Verification items for the finished model (mm, model axes). Face numbers are marked on the shaded views. A direction names the side the tool comes from. Coordinates: 2 decimals unless noted, no trailing zeros. Order: outer loops, then holes, each group sorted by start corner. A loop starts at its lowest first (then second) coordinate and runs counter-clockwise, first axis right, second up. Notation, with made-up numbers: M 70,7 L 115,7 A9 ccw 115,20 Z; hole C -32.75,19.5 d5. An arc over 180 degrees is marked long. Use one line per item in the form item = value. Start each with the question number.
```python
from build123d import *
from build123d.topology import SkipClean

# Parameters (mm, degrees)
BASE_EXTRUDE_DEPTH  = 5.76
SKETCH2_R           = 2.65
BOSS_EXTRUDE1_DEPTH = 9.45
CUT_EXTRUDE3_DEPTH  = 53.449290987
SKETCH4_R           = 1.37
BOSS_EXTRUDE2_DEPTH = 2.64
BOSS_EXTRUDE2_DRAFT = -1
SKETCH7_R           = 1.15
CUT_EXTRUDE4_DEPTH  = 11.09
CUT_EXTRUDE5_DEPTH  = 53.988618848
CUT_EXTRUDE6_START  = -3.76
CUT_EXTRUDE6_DEPTH  = 3.76
BOSS_EXTRUDE3_DEPTH = 1.65
SKETCH11_W          = 10.1
SKETCH11_H          = 3.76
CUT_EXTRUDE7_DEPTH  = 1.5
SKETCH12_W          = 10.1
SKETCH12_H          = 1.65
CUT_EXTRUDE8_DEPTH  = 1.5
BOSS_EXTRUDE4_DEPTH = 3.76
FILLET1_R           = 0.7
BOSS_EXTRUDE5_START = -3.76
BOSS_EXTRUDE5_DEPTH = 5.18
FILLET5_R           = 0.685
BOSS_EXTRUDE6_DEPTH = 3.48
BOSS_EXTRUDE7_START = -1.26
BOSS_EXTRUDE7_DEPTH = 1.26
BOSS_EXTRUDE8_DEPTH = 4
SKETCH18_W          = 2
SKETCH18_H          = 4.75
CUT_EXTRUDE9_DEPTH  = 48.255056695
FILLET2_R           = 1
SKETCH21_R          = 1.46
CUT_EXTRUDE13_DEPTH = 6.58


with BuildPart() as part:
    # Sketch1 → Base-Extrude (new body)
    with BuildSketch(Plane.XY):
        with BuildLine():
            Line((0, 0), (17.107264567, 14.875))
            Line((17.107264567, 14.875), (47.107264567, 14.875))
            ThreePointArc((47.107264567, 14.875), (49.4, 0), (47.107264567, -14.875))
            Line((47.107264567, -14.875), (17.107264567, -14.875))
            Line((17.107264567, -14.875), (0, 0))
        make_face()
    extrude(amount=BASE_EXTRUDE_DEPTH)

    # Sketch2 → Boss-Extrude1 (add)
    with BuildSketch(Plane.XY.offset(5.76)):
        with Locations((4.038670317, 0)):
            Circle(SKETCH2_R)
    extrude(amount=-BOSS_EXTRUDE1_DEPTH)

    # Sketch3 → Cut-Extrude3 (cut, through all)
    with SkipClean():  # the faces are left unmerged after this step: merging them gives an invalid solid
        with BuildSketch(Plane.XY.offset(5.76)):
            with BuildLine():
                Line((0, 0), (2.299855448, -1.999755698))
                ThreePointArc((2.299855448, -1.999755698), (1.388670317, 0), (2.299855448, 1.999755698))
                Line((2.299855448, 1.999755698), (0, 0))
            make_face()
        extrude(amount=-CUT_EXTRUDE3_DEPTH, mode=Mode.SUBTRACT)


with BuildPart() as boss_extrude2_tool:
    # Sketch4 → Boss-Extrude2 (with draft: the straight prism first)
    with BuildSketch(Plane(origin=(0, 0, -3.69), x_dir=(-1, 0, 0), z_dir=(0, 0, -1))):
        with Locations((-4.038670317, 0)):
            Circle(SKETCH4_R)
    extrude(amount=BOSS_EXTRUDE2_DEPTH)
    # Boss-Extrude2: the draft: its side faces are tilted about the plane it starts from
    boss_extrude2_sides = [boss_extrude2_tool.faces().sort_by_distance(p)[0] for p in [
        (5.408670317, 0, -5.01),
    ]]
    draft(boss_extrude2_sides, Plane(origin=(0, 0, -3.69), x_dir=(-1, 0, 0), z_dir=(0, 0, -1)), BOSS_EXTRUDE2_DRAFT)


with BuildPart() as part_1:
    add(part.part)

    # Boss-Extrude2: add boss_extrude2_tool
    add(boss_extrude2_tool.part)

    # Sketch7 → Cut-Extrude4 (cut)
    with SkipClean():  # the faces are left unmerged after this step: merging them gives an invalid solid
        with BuildSketch(Plane.XY.offset(5.76)):
            with Locations((3.701631462, 0)):
                Circle(SKETCH7_R)
        extrude(amount=-CUT_EXTRUDE4_DEPTH, mode=Mode.SUBTRACT)

    # Sketch8 → Cut-Extrude5 (cut, through all)
    with SkipClean():  # the faces are left unmerged after this step: merging them gives an invalid solid
        with BuildSketch(Plane.XY.offset(5.76)):
            Polygon((15.128209475, 1.37), (42.128209475, 1.37), (42.128209475, -1.63), (39.528209475, -1.63), (37.70423163, -8.90482679), (17.334716619, -3.797688825), (17.878209475, -1.63), (15.128209475, -1.63), align=None)
        extrude(amount=-CUT_EXTRUDE5_DEPTH, mode=Mode.SUBTRACT)

    # Sketch9 → Cut-Extrude6 (cut)
    with SkipClean():  # the faces are left unmerged after this step: merging them gives an invalid solid
        with BuildSketch(Plane(origin=(0, 0, 0), x_dir=(-1, 0, 0), z_dir=(0, 0, -1)).offset(CUT_EXTRUDE6_START)):
            with BuildLine():
                Line((-5.085732276, 2.434370813), (-17.66820206, 13.375))
                Line((-17.66820206, 13.375), (-45.994775519, 13.375))
                ThreePointArc((-45.994775519, 13.375), (-47.9, 0), (-45.994775519, -13.375))
                Line((-45.994775519, -13.375), (-17.66820206, -13.375))
                Line((-17.66820206, -13.375), (-5.085732276, -2.434370813))
                ThreePointArc((-5.085732276, -2.434370813), (-6.688670317, 0), (-5.085732276, 2.434370813))
            make_face()
        extrude(amount=CUT_EXTRUDE6_DEPTH, mode=Mode.SUBTRACT)

    # Sketch10 → Boss-Extrude3 (add)
    with SkipClean():  # the faces are left unmerged after this step: merging them gives an invalid solid
        with BuildSketch(Plane(origin=(0, 0, 3.76), x_dir=(-1, 0, 0), z_dir=(0, 0, -1))):
            Polygon((-43.128209475, -2.63), (-43.128209475, 2.37), (-14.128209475, 2.37), (-14.128209475, -2.63), (-16.59653252, -2.63), (-16.121542667, -4.524468684), (-38.431011489, -10.118000741), (-40.308437282, -2.63), align=None)
            Polygon((-15.128209475, 1.37), (-15.128209475, -1.63), (-17.878209475, -1.63), (-17.334716619, -3.797688825), (-37.70423163, -8.90482679), (-39.528209475, -1.63), (-42.128209475, -1.63), (-42.128209475, 1.37), align=None, mode=Mode.SUBTRACT)
        extrude(amount=BOSS_EXTRUDE3_DEPTH)

    # Sketch11 → Cut-Extrude7 (cut)
    with SkipClean():  # the faces are left unmerged after this step: merging them gives an invalid solid
        with BuildSketch(Plane(origin=(0, 14.875, 0), x_dir=(-1, 0, 0), z_dir=(0, 1, 0))):
            with Locations((-27.157264567, 1.88)):
                Rectangle(SKETCH11_W, SKETCH11_H)
        extrude(amount=-CUT_EXTRUDE7_DEPTH, mode=Mode.SUBTRACT)

    # Sketch12 → Cut-Extrude8 (cut)
    with BuildSketch(Plane.XZ.offset(14.875)):
        with Locations((27.157264567, 0.825)):
            Rectangle(SKETCH12_W, SKETCH12_H)
    extrude(amount=-CUT_EXTRUDE8_DEPTH, mode=Mode.SUBTRACT)

    # Sketch13 → Boss-Extrude4 (add)
    with BuildSketch(Plane(origin=(0, 0, 3.76), x_dir=(-1, 0, 0), z_dir=(0, 0, -1))):
        Polygon((-18.37820206, -13.375), (-18.37820206, -9.095), (-16.95820206, -9.095), (-16.95820206, -12.757645311), (-17.66820206, -13.375), align=None)
    extrude(amount=BOSS_EXTRUDE4_DEPTH)

    # Fillet1
    fillet1_edges = [part_1.edges().sort_by_distance(p)[0] for p in [
        (16.95820206, -9.095, 1.88),
        (18.37820206, -9.095, 1.88),
    ]]
    fillet(fillet1_edges, radius=FILLET1_R)

    # Sketch14 → Boss-Extrude5 (add)
    with BuildSketch(Plane(origin=(0, 0, 0), x_dir=(-1, 0, 0), z_dir=(0, 0, -1)).offset(BOSS_EXTRUDE5_START)):
        Polygon((-38.431011489, -10.675), (-39.801011489, -10.675), (-39.801011489, -13.375), (-45.994775519, -13.375), (-47.107264567, -14.875), (-38.431011489, -14.875), align=None)
    extrude(amount=BOSS_EXTRUDE5_DEPTH)

    # Fillet5
    fillet5_edges = [part_1.edges().sort_by_distance(p)[0] for p in [
        (38.431011489, -10.675, 1.17),
        (39.801011489, -10.675, 1.17),
    ]]
    fillet(fillet5_edges, radius=FILLET5_R - 0.0001)  # a hair under: the kernel refuses the full size

    # Sketch15 → Boss-Extrude6 (add)
    with BuildSketch(Plane(origin=(0, 0, 0), x_dir=(-1, 0, 0), z_dir=(0, 0, -1))):
        with BuildLine():
            Line((-47.107264567, 14.875), (-45.53179521, 14.875))
            ThreePointArc((-45.53179521, 14.875), (-47.9, 0), (-45.53179521, -14.875))
            Line((-45.53179521, -14.875), (-47.107264567, -14.875))
            ThreePointArc((-47.107264567, -14.875), (-49.4, 0), (-47.107264567, 14.875))
        make_face()
    extrude(amount=BOSS_EXTRUDE6_DEPTH)

    # Sketch16 → Boss-Extrude7 (add)
    with BuildSketch(Plane(origin=(0, 0, -3.48), x_dir=(-1, 0, 0), z_dir=(0, 0, -1)).offset(BOSS_EXTRUDE7_START)):
        with BuildLine():
            Line((-47.107264567, -14.875), (-45.53179521, -14.875))
            ThreePointArc((-45.53179521, -14.875), (-46.189233829, -12.687185592), (-46.741612583, -10.470513507))
            Line((-46.741612583, -10.470513507), (-55.921612583, -10.470513507))
            Line((-55.921612583, -10.470513507), (-53.33179521, -14.875))
            Line((-53.33179521, -14.875), (-47.107264567, -14.875))
        make_face()
        with BuildLine():
            Line((-47.107264567, 14.875), (-45.53179521, 14.875))
            ThreePointArc((-45.53179521, 14.875), (-46.189233829, 12.687185592), (-46.741612583, 10.470513507))
            Line((-46.741612583, 10.470513507), (-55.921612583, 10.470513507))
            Line((-55.921612583, 10.470513507), (-53.33179521, 14.875))
            Line((-53.33179521, 14.875), (-47.107264567, 14.875))
        make_face()
    extrude(amount=BOSS_EXTRUDE7_DEPTH)

    # Sketch17 → Boss-Extrude8 (add)
    with BuildSketch(Plane.XY.offset(5.76)):
        Polygon((45.907264567, 14.875), (45.907264567, 17.765), (49.007264567, 17.765), (49.007264567, 19.625), (43.907264567, 19.625), (43.907264567, 14.875), align=None)
    extrude(amount=-BOSS_EXTRUDE8_DEPTH)

    # Sketch18 → Cut-Extrude9 (cut, through all)
    with BuildSketch(Plane.ZY.offset(-43.907264567)):
        with Locations((4.76, 17.25)):
            Rectangle(SKETCH18_W, SKETCH18_H)
    extrude(amount=-CUT_EXTRUDE9_DEPTH, mode=Mode.SUBTRACT)

    # Fillet2
    fillet2_edges = [part_1.edges().sort_by_distance(p)[0] for p in [
        (45.907264567, 17.765, 2.76),
    ]]
    fillet(fillet2_edges, radius=FILLET2_R)

    # Sketch21 → Cut-Extrude13 (cut)
    with BuildSketch(Plane(origin=(0, 0, 1.18), x_dir=(-1, 0, 0), z_dir=(0, 0, -1))):
        with Locations(Location((-3.701631462, 0, 0), (0, 0, 90))):
            Circle(SKETCH21_R)
    extrude(amount=-CUT_EXTRUDE13_DEPTH, mode=Mode.SUBTRACT)


solid = part_1.part
```
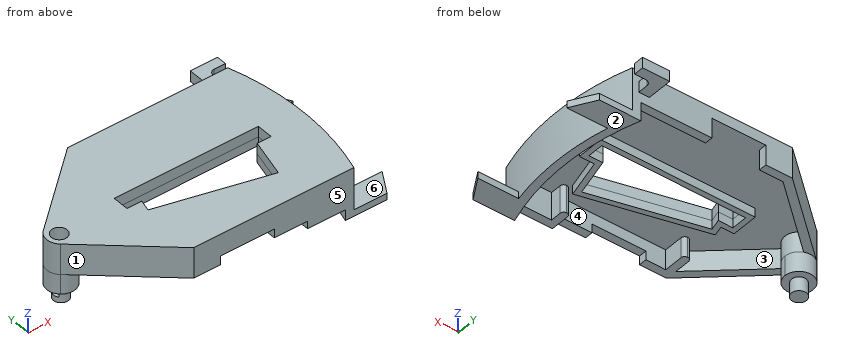
1. Depth check by flat-ended pin: P1, Ø6, axis at y = -4, z = -1, coming from the -X side; P2, Ø1.4, axis at x = 46, y = 16.5, coming from the +Z side; P3, Ø1, axis at x = 41.5, z = 4.5, coming from the +Y side (3 decimals); P4, Ø2, axis at x = 18, y = -1, coming from the +Z side. Enter the tip coordinate at first touch or a pass-through.
2. Cross-section at A-A on x = 50.5. Enter the section's corners in (y, z) (3 decimals), and give its area (3 significant figures).
3. Tool access check on the marked faces 4, 5 and 6. Record the directions out of +Z, -Z, +X, -X, +Y, -Y that give a thin tool (end or side, any length) a straight path to the whole face; none if there is none.
4. Material ranges on line 1 along X through (y, z) = (0, 4.1); line 2 along X through (y, z) = (0, -0.5); line 3 along Y through (x, z) = (35.5, 1.75) (3 decimals), recorded low to high.
5. Cross-section at C-C on x = 24. Enter the section's corners in (y, z) (3 decimals).
6. Cross-section at B-B on y = 6.5. Enter the section's corners in (x, z), and give its area (3 significant figures).
7. Cross-section at D-D on x = 35. Enter the section's corners in (y, z) (3 decimals).
8. Release check for a two-part mould opening along X. For the marked faces 1, 2 and 3 record: pulls with the +X half, pulls with the -X half, needs draft (parallel to the pull), parting line crosses it, or undercut.
Final values:
q1.P1 = 1.58
q1.P2 = 3.76
q1.P3 = 14.875
q1.P4 = 5.76
q2.outline = M -14.875,-3.48 L -10.471,-3.48 L -10.471,-2.22 L -14.875,-2.22 Z; M 10.471,-3.48 L 14.875,-3.48 L 14.875,-2.22 L 10.471,-2.22 Z
q2.area = 11.1 mm2
q3.face_4 = -Z
q3.face_5 = +Z, -Z, +X, -X, -Y
q3.face_6 = +Z, +X, -Y
q4.line_1 = 1.39 to 2.24, 5.16 to 15.13, 42.13 to 49.4
q4.line_2 = 1.39 to 2.55, 4.85 to 6.69, 47.9 to 49.4
q4.line_3 = -14.875 to -13.375, 13.375 to 14.875
q5.outline = M -14.875,1.65 L -13.375,1.65 L -13.375,3.76 L -6.5,3.76 L -6.5,2.11 L -5.469,2.11 L -5.469,5.76 L -14.875,5.76 Z; M 1.37,2.11 L 2.37,2.11 L 2.37,3.76 L 14.875,3.76 L 14.875,5.76 L 1.37,5.76 Z
q6.outline = M 7.48,0 L 9.76,0 L 9.76,3.76 L 47.46,3.76 L 47.46,-3.48 L 48.97,-3.48 L 48.97,5.76 L 7.48,5.76 Z
q6.area = 103 mm2
q7.outline = M -14.875,0 L -13.375,0 L -13.375,3.76 L -9.258,3.76 L -9.258,2.11 L -8.227,2.11 L -8.227,5.76 L -14.875,5.76 Z; M 1.37,2.11 L 2.37,2.11 L 2.37,3.76 L 13.375,3.76 L 13.375,0 L 14.875,0 L 14.875,5.76 L 1.37,5.76 Z
q8.face_1 = pulls with the -X half
q8.face_2 = needs draft
q8.face_3 = undercut
